Autodesk Inventor part; units mm, degrees
ref_plane "YZ Plane" through (0, 0, 0) normal (1, 0, 0) x (0, 1, 0)
ref_plane "XZ Plane" through (0, 0, 0) normal (0, 1, 0) x (-1, 0, 0)
ref_plane "XY Plane" through (0, 0, 0) normal (0, 0, 1) x (1, 0, 0)
sketch "Sketch1" plane through (0, 0, 0) normal (0, 1, 0) x (-1, 0, 0)
  circle A0 centre (0, 0) radius 225.425
  dimension "d0" = 450.85
extrude "Extrusion1" add sketch "Sketch1" along normal blind 12.7
sketch "Sketch2" plane through (0, 12.7, 0) normal (0, 1, 0) x (1, 0, 0)
  circle A0 centre (0, 0) radius 225.425
  circle A1 centre (0, 12.7) radius 6.35
  dimension "d3" = 12.7
  dimension "d4" = 12.7
extrude "Extrusion2" cut sketch "Sketch2" against normal blind 12.7 contours A1
pattern_circular "Circular Pattern1" count 4 over 360 about axis through (0, -10, 0) along (0, 1, 0) of "Extrusion2"
sketch "Sketch3" plane through (0, 12.7, 0) normal (0, 1, 0) x (1, 0, 0)
  circle A0 centre (0, 0) radius 225.425
  line L0 (-38.1, 38.1) -> (38.1, 38.1)
  line L1 (38.1, 38.1) -> (38.1, -38.1)
  line L2 (38.1, -38.1) -> (-38.1, -38.1)
  line L3 (-38.1, -38.1) -> (-38.1, 38.1)
  circle A1 centre (-31.75, 31.75) radius 1.5875
  circle A2 centre (31.75, 31.75) radius 1.5875
  circle A3 centre (-31.75, -31.75) radius 1.5875
  circle A4 centre (31.75, -31.75) radius 1.5875
  line L4 (-63.5, 63.5) -> (63.5, 63.5)
  line L5 (63.5, 63.5) -> (63.5, -63.5)
  line L6 (63.5, -63.5) -> (-63.5, -63.5)
  line L7 (-63.5, -63.5) -> (-63.5, 63.5)
  circle A5 centre (53.975, 53.975) radius 3.175
  circle A6 centre (-53.975, 53.975) radius 3.175
  circle A7 centre (53.975, -53.975) radius 3.175
  circle A8 centre (-53.975, -53.975) radius 3.175
  circle A9 centre (150.495, 0) radius 6.35
  circle A10 centre (-75.2475, 130.3325) radius 6.35
  circle A11 centre (-75.2475, -130.3325) radius 6.35
  dimension "d10" = 76.2
  dimension "d11" = 76.2
  dimension "d12" = 38.1
  dimension "d13" = 38.1
  dimension "d14" = 3.175
  dimension "d15" = 6.35
  dimension "d16" = 6.35
  dimension "d19" = 63.5
  dimension "d22" = 63.5
  dimension "d27" = 127
  dimension "d28" = 127
  dimension "d29" = 63.5
  dimension "d30" = 63.5
  dimension "d31" = 6.35
  dimension "d32" = 9.525
  dimension "d33" = 9.525
  dimension "d36" = 107.95
  dimension "d39" = 107.95
  dimension "d42" = 12.7
  dimension "d43" = 150.495
  dimension "d46" = 360
extrude "Extrusion3" cut sketch "Sketch3" against normal blind 12.7 contours A1 | A2 | A3 | A4 | A5 | A6 | A7 | A8 | A9 | A10 | A11
properties part number "Base_Can"
The listing builds one solid part. Answer for the finished solid, in the listing's coordinates (mm). Coordinates: 2 decimals unless noted, no trailing zeros. Order: outer loops, then holes, each group sorted by start corner. A loop starts at its lowest first (then second) coordinate and runs counter-clockwise, first axis right, second up. Notation, with made-up numbers: (17, 81) -> (59, 81) arc R24 ccw to (59, 100) -> close; hole circle Ø8 at (86.5, -5). An arc over 180 degrees is marked (long way). Answer in a Markdown table with one row per item. Add a question column.
Item 1: Determine the mould class of faces 1 (the face through (225.207, 6.261, -9.912)), 2 (the face through (3, 0, 3)), 3 (the face through (3.414, 6.439, -18.054)) for opening direction Z: +Z half, -Z half, draft (parallel to the pull), parting line (faces both ways), or undercut.
Item 2: Find section C-C (x = 12.7). Write down the section's boundary in (y, z).
Item 3: Each of these flat-tipped pins is pushed along its axis until it touches: P1, Ø14.5, axis at x = 150.495, z = 0, coming from the +Y side; P2, Ø6, axis at x = 179.5, y = 3.5, coming from the +Z side; P3, Ø6, axis at x = 125, y = 9, coming from the -Z side; P4, Ø4, axis at y = 4.5, z = -99.5, coming from the +X side. Where does it stop, or does it pass through?
Item 4: Find section D-D (x = -109.5). Write down the section's boundary in (y, z), then the cut area to 3 significant figures.
Item 5: Find section B-B (y = 4). State how many separate pieces and enclosed holes the cut face has, then the cut area to 3 significant figures.
Item 6: Find the intervals of material crossed by L1, parallel to Z at x = 0, y = 8.5 (3 decimals); L2, parallel to Z at x = -78.5, y = 7; L3, parallel to X at y = 4.75, z = 31.75, in increasing order. Write a range as from..to.
Item 7: Find section A-A (z = 0). Write down the section's boundary in (x, y) (3 decimals), then the cut area to 3 significant figures.
Result set:
| question | item | result |
|---|---|---|
| 1 | face 1 | parting line |
| 1 | face 2 | draft |
| 1 | face 3 | undercut |
| 2 | outline | (0, -225.07) -> (12.7, -225.07) -> (12.7, -6.35) -> (0, -6.35) -> close; (0, 6.35) -> (12.7, 6.35) -> (12.7, 225.07) -> (0, 225.07) -> close |
| 3 | P1 | stops at y = 12.7 |
| 3 | P2 | stops at z = 140.23 |
| 3 | P3 | stops at z = -189.56 |
| 3 | P4 | stops at x = 203.25 |
| 4 | outline | (0, -197.04) -> (12.7, -197.04) -> (12.7, 197.04) -> (0, 197.04) -> close |
| 4 | area | 5,000 mm² |
| 5 | separate pieces | 1 |
| 5 | enclosed holes | 15 |
| 5 | area | 159,000 mm² |
| 6 | L1 | z = -225.425..-19.05, -6.35..6.35, 19.05..225.425 |
| 6 | L2 | z = -211.32..-135.79, -124.88..124.88, 135.79..211.32 |
| 6 | L3 | x = -223.18..-33.34, -30.16..30.16, 33.34..223.18 |
| 7 | outline | (-225.425, 0) -> (-19.05, 0) -> (-19.05, 12.7) -> (-225.425, 12.7) -> close; (-6.35, 0) -> (6.35, 0) -> (6.35, 12.7) -> (-6.35, 12.7) -> close; (19.05, 0) -> (144.145, 0) -> (144.145, 12.7) -> (19.05, 12.7) -> close; (156.845, 0) -> (225.425, 0) -> (225.425, 12.7) -> (156.845, 12.7) -> close |
| 7 | area | 5,240 mm² |
